Input: part model. Units: mm. Frame: model coordinates. A direction names the side the tool comes from. Give positions to 0.01 mm unless a question says otherwise; leave off trailing zeros. Order: outer loops, then holes, each group sorted by start corner. A loop starts at its lowest first (then second) coordinate and runs counter-clockwise, first axis right, second up. Notation, with made-up numbers: M -15.5,5.25 L 8.5,5.25 A16 cw 8.5,23.25 Z; hole C 1,-26.75 d8. An arc over 180 degrees is marked long. Use a Markdown table: item, result.
from build123d import *

# Parameters (mm, degrees)
BOSS_EXTRUDE1_DEPTH = 3.175
FILLET1_R           = 3.175
SKETCH2_R           = 1.5875
CUT_EXTRUDE1_DEPTH  = 16.165203955
SKETCH3_R           = 0.127
CUT_EXTRUDE2_DEPTH  = 0.254
CUT_EXTRUDE3_START  = -0.254
SKETCH4_R           = 0.127
CUT_EXTRUDE3_DEPTH  = 0.254
SKETCH5_W           = 0.508
SKETCH5_H           = 0.508
BOSS_EXTRUDE2_DEPTH = 8.89
SKETCH6_W           = 0.508
SKETCH6_H           = 0.508
BOSS_EXTRUDE3_DEPTH = 1.27


with BuildPart() as part:
    # Sketch1 → Boss-Extrude1 (new, symmetric)
    with BuildSketch(Plane.XY):
        Polygon((12.319, 0), (-12.319, 0), (-12.319, 2.54), (-6.1595, 2.54), (-6.1595, 10.795), (-1.5875, 10.795), (-1.5875, 2.032), (1.5875, 2.032), (1.5875, 10.795), (6.1595, 10.795), (6.1595, 2.54), (12.319, 2.54), align=None)
    extrude(amount=BOSS_EXTRUDE1_DEPTH, both=True)

    # Fillet1
    fillet1_edges = [part.edges().sort_by_distance(p)[0] for p in [
        (-12.319, 1.27, 3.175),
        (-12.319, 1.27, -3.175),
        (12.319, 1.27, -3.175),
        (12.319, 1.27, 3.175),
    ]]
    fillet(fillet1_edges, radius=FILLET1_R - 0.0001)  # a hair under: the kernel refuses the full size

    # Sketch2 → Cut-Extrude1 (cut, through all)
    with BuildSketch(Plane(origin=(0, 2.54, 0), x_dir=(1, 0, 0), z_dir=(0, 1, 0))):
        with Locations(Location((-9.525, 0, 0), (0, 0, 270))):
            Circle(SKETCH2_R)
        with Locations(Location((9.525, 0, 0), (0, 0, 270))):
            Circle(SKETCH2_R)
    extrude(amount=-CUT_EXTRUDE1_DEPTH, mode=Mode.SUBTRACT)

    # Sketch3 → Cut-Extrude2 (cut)
    with BuildSketch(Plane.ZY.offset(-1.5875)):
        with Locations(Location((0, 8.001, 0), (0, 0, 270))):
            Circle(SKETCH3_R)
    extrude(amount=-CUT_EXTRUDE2_DEPTH, mode=Mode.SUBTRACT)

    # Sketch4 → Cut-Extrude3 (cut)
    with BuildSketch(Plane(origin=(-1.5875, 0, 0), x_dir=(0, 0, -1), z_dir=(1, 0, 0)).offset(CUT_EXTRUDE3_START)):
        with Locations(Location((0, 8.001, 0), (0, 0, 270))):
            Circle(SKETCH4_R)
    extrude(amount=CUT_EXTRUDE3_DEPTH, mode=Mode.SUBTRACT)

    # Sketch5 → Boss-Extrude2 (add)
    with BuildSketch(Plane.XZ):
        with Locations((-4.064, 1.27)):
            Rectangle(SKETCH5_W, SKETCH5_H)
        with Locations((-4.064, -1.27)):
            Rectangle(SKETCH5_W, SKETCH5_H)
        with Locations((4.064, 1.905)):
            Rectangle(SKETCH5_W, SKETCH5_H)
        with Locations((4.064, 0)):
            Rectangle(SKETCH5_W, SKETCH5_H)
        with Locations((4.064, -1.905)):
            Rectangle(SKETCH5_W, SKETCH5_H)
    extrude(amount=BOSS_EXTRUDE2_DEPTH)

    # Sketch6 → Boss-Extrude3 (add)
    with BuildSketch(Plane.XZ.offset(8.89)):
        with Locations((-4.064, -1.27)):
            Rectangle(SKETCH6_W, SKETCH6_H)
    extrude(amount=BOSS_EXTRUDE3_DEPTH)


solid = part.part
1) First-contact query: pin 1 Ø0.6 at (x, z) = (4, 0) entering from -Y; pin 2 Ø2 at (y, z) = (-5, -1) entering from +X; pin 3 Ø3 at (x, z) = (9, -0.5) entering from -Y. Flat tips, straight axial feed; report the tip coordinate or a pass-through.
Response values:
| item | result |
|---|---|
| pin 1 | stops at y = -8.89 |
| pin 2 | stops at x = 4.32 |
| pin 3 | stops at y = 0 |
2) Cut plane B-B on x = 10.5. Return loops of the section in (y, z).
Response values:
| item | result |
|---|---|
| outline | M 0,-2.87 L 2.54,-2.87 L 2.54,-1.25 L 0,-1.25 Z; M 0,1.25 L 2.54,1.25 L 2.54,2.87 L 0,2.87 Z |
3) Cut plane C-C on z = 2.75. Return loops of the section in (x, y) (1 decimal).
Response values:
| item | result |
|---|---|
| outline | M -10.7,0 L 10.7,0 L 10.7,2.5 L 6.2,2.5 L 6.2,10.8 L 1.6,10.8 L 1.6,2 L -1.6,2 L -1.6,10.8 L -6.2,10.8 L -6.2,2.5 L -10.7,2.5 Z |
4) Reachability of faces 1 (the face through (8, 2.54, -1)), 2 (the face through (-1.588, 6, 0)), 3 (the face through (-6.16, 7, 0)) from +Z, -Z, +X, -X, +Y, -Y: full face, straight path, thin tool, end or side. Return the list, or none.
Response values:
| item | result |
|---|---|
| face 1 | +Z, -Z, +X, +Y |
| face 2 | +Z, -Z, +Y |
| face 3 | +Z, -Z, -X, +Y |
5) Mould query, pull axis X, two halves, no side actions, for faces 4 (the face through (0, 0, 0)), 5 (the face through (-9, 1.3, 1.5)), 6 (the face through (11.364, 1.252, -2.27)). Classes: released by +X, released by -X, zero draft, split by the parting line, or undercut.
Response values:
| item | result |
|---|---|
| face 4 | zero draft |
| face 5 | undercut |
| face 6 | released by +X |
6) Cut plane A-A on y = -5. Return loops of the section in (x, z).
Response values:
| item | result |
|---|---|
| outline | M -4.32,-1.52 L -3.81,-1.52 L -3.81,-1.02 L -4.32,-1.02 Z; M -4.32,1.02 L -3.81,1.02 L -3.81,1.52 L -4.32,1.52 Z; M 3.81,-2.16 L 4.32,-2.16 L 4.32,-1.65 L 3.81,-1.65 Z; M 3.81,-0.25 L 4.32,-0.25 L 4.32,0.25 L 3.81,0.25 Z; M 3.81,1.65 L 4.32,1.65 L 4.32,2.16 L 3.81,2.16 Z |
7) Material intervals for line 1 (X direction, y = 1.9, z = 0); line 2 (X direction, y = 7.5, z = -2.75); line 3 (Y direction, x = -6.25, z = -1), sorted ascending. Write a range as from..to.
Response values:
| item | result |
|---|---|
| line 1 | x = -12.32..-11.11, -7.94..7.94, 11.11..12.32 |
| line 2 | x = -6.16..-1.59, 1.59..6.16 |
| line 3 | y = 0..2.54 |
8) Cut plane D-D on x = 0. Return loops of the section in (y, z) (3 decimals).
Response values:
| item | result |
|---|---|
| outline | M 0,-3.175 L 2.032,-3.175 L 2.032,3.175 L 0,3.175 Z |
